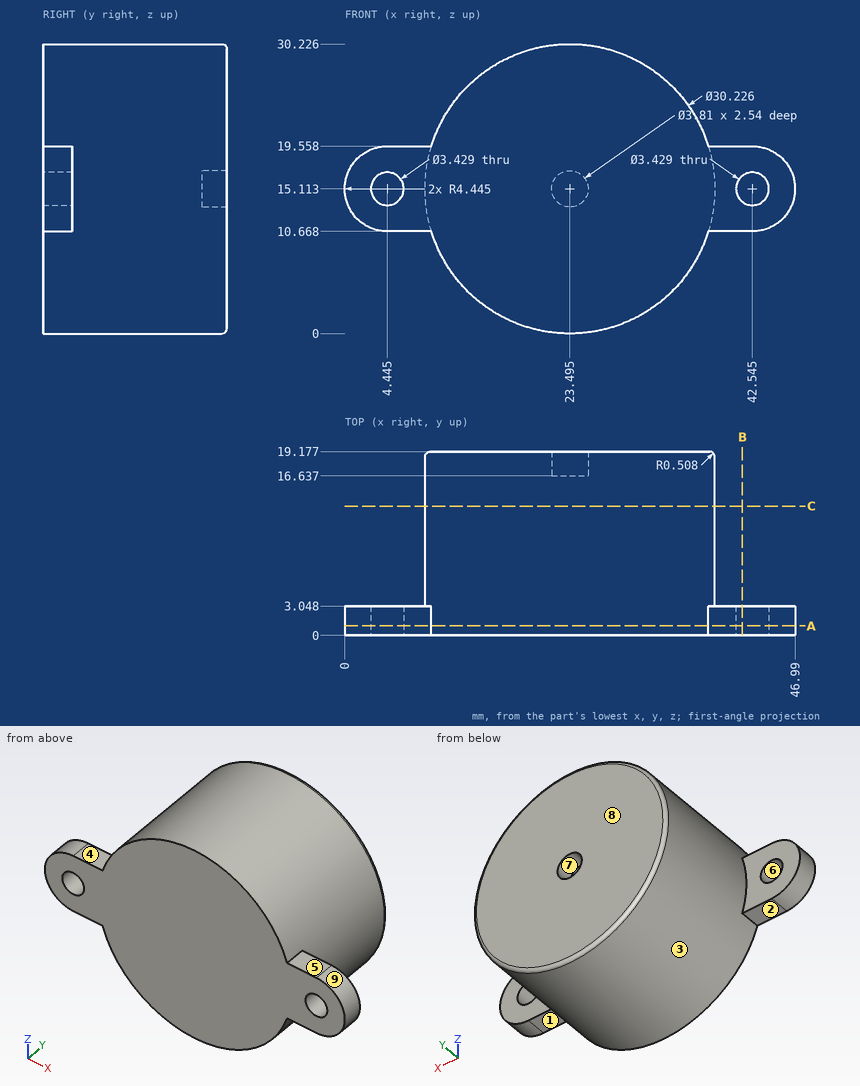
Check sheet for the drawn part. Datum: minimum x, y, z corner. Units: mm. A direction names the side the tool comes from. Coordinates: 2 decimals unless noted, no trailing zeros. Write each loop counter-clockwise with the first axis right and the second up, starting at its lowest first coordinate (ties: lowest second). Pieces come first, ordered by that corner, then holes. Notation, with made-up numbers: (-30.5, 6.5) - (-9.5, 6.5) arc R20 cw to (-9.5, 42.5) - close; hole circle Ø3 at (-32, 88.25). An arc over 180 degrees is marked (long way). Answer as a JSON object with one key per item and string values.
(1) Cross-section at C-C on y = 13.5. Record the cut outline in (x, z) (3 decimals).
Report:
{"outline": "circle Ø30.226 at (23.495, 15.113)"}
(2) Gauge pin test, flat ends, axial feed: pin 1 Ø3 at (x, y) = (9, 15) entering from +Z; pin 2 Ø4 at (x, z) = (4.445, 15.113) entering from +Y; pin 3 Ø2.5 at (x, y) = (6, 1.5) entering from +Z. Record the tip position at first contact, or that the pin passes through.
Report:
{"pin 1": "z = 22.83", "pin 2": "y = 3.05", "pin 3": "z = 19.56"}
(3) Cross-section at B-B on x = 41.5. Record the cut outline in (y, z), plus the area to 3 significant figures.
Report:
{"outline": "(0, 10.67) - (3.05, 10.67) - (3.05, 13.75) - (0, 13.75) - close; (0, 16.47) - (3.05, 16.47) - (3.05, 19.56) - (0, 19.56) - close", "area": "18.8 mm^2"}
(4) Tool access check on the marked faces 1, 2, 3, 4 and 5. Record the directions out of +Z, -Z, +X, -X, +Y, -Y that give a thin tool (end or side, any length) a straight path to the whole face; none if there is none.
Report:
{"face 1": "-Z, +X, +Y, -Y", "face 2": "-Z, -X, +Y, -Y", "face 3": "+Y", "face 4": "+Z, -X, +Y, -Y", "face 5": "+Z, +X, +Y, -Y"}
(5) Mould release check, pull along X, two halves, no side actions. Record for the marked faces 6, 7, 8 and 9: pulls with the +X half, pulls with the -X half, needs draft (parallel to the pull), parting line crosses it, or undercut.
Report:
{"face 6": "undercut", "face 7": "undercut", "face 8": "needs draft", "face 9": "pulls with the +X half"}
(6) Cross-section at A-A on y = 1. Record the cut outline in (x, z) (1 decimal), plus the area to 3 significant figures.
Report:
{"outline": "(4.4, 10.7) - (9.1, 10.7) arc R15.1 ccw to (37.9, 10.7) - (42.5, 10.7) arc R4.4 ccw to (42.5, 19.6) - (37.9, 19.6) arc R15.1 ccw to (9.1, 19.6) - (4.4, 19.6) arc R4.4 ccw to start; hole circle Ø3.4 at (4.4, 15.1); hole circle Ø3.4 at (42.5, 15.1)", "area": "835 mm^2"}
(7) Thickness scan on line 1 along Y through (x, z) = (7, 11); line 2 along Z through (x, y) = (33, 11); line 3 along Z through (x, y) = (3, 2.25). Record the ranges inside material, lowest first.
Report:
{"line 1": "0 to 3.05", "line 2": "3.36 to 26.86", "line 3": "10.91 to 14.19, 16.04 to 19.32"}
